from build123d import *

# Parameters (mm, degrees)
SKETCH1_W               = 21
SKETCH1_H               = 9
BOSS_EXTRUDE1_DEPTH     = 4
CUT_EXTRUDE1_REACH      = 15.946
SKETCH2_W               = 17
SKETCH2_H               = 7
CUT_EXTRUDE3_REACH      = 15.946
SKETCH5_W               = 2
SKETCH5_H               = 9
BOSS_EXTRUDE2_REACH     = 21.931
SKETCH9_W               = 2
SKETCH9_H               = 3
BOSS_EXTRUDE3_DEPTH     = 8
SKETCH11_W              = 3
SKETCH11_H              = 5
BOSS_EXTRUDE4_DEPTH     = 11.25
BOSS_EXTRUDE5_START     = -4
BOSS_EXTRUDE5_OUTLINE_W = 3
BOSS_EXTRUDE5_OUTLINE_H = 5
BOSS_EXTRUDE5_DEPTH     = 8
SKETCH13_R              = 0.75
CUT_EXTRUDE4_DEPTH      = 2.5
BOSS_EXTRUDE6_DEPTH     = 5
BOSS_EXTRUDE7_REACH     = 29.795


# Read off the part's stored shape, not the designer's step: Boss-Extrude5
with BuildPart() as part:
    # Sketch1 → Boss-Extrude1 (new, symmetric)
    with BuildSketch(Plane.XY):
        Rectangle(SKETCH1_W, SKETCH1_H)
    extrude(amount=BOSS_EXTRUDE1_DEPTH, both=True)

    # Sketch2 → Cut-Extrude1 (cut, up to next)
    with BuildSketch(Plane.XY.offset(4), mode=Mode.PRIVATE) as cut_extrude1_sk1:
        with Locations((0, -1)):
            Rectangle(SKETCH2_W, SKETCH2_H)
    cut_extrude1_tool1 = extrude(cut_extrude1_sk1.sketch, amount=-CUT_EXTRUDE1_REACH, mode=Mode.PRIVATE) & part.part
    add(cut_extrude1_tool1.solids().sort_by_distance((0, -1, 4))[0], mode=Mode.SUBTRACT)

    # Sketch5 → Cut-Extrude3 (cut, up to next)
    with BuildSketch(Plane.XY.offset(4), mode=Mode.PRIVATE) as cut_extrude3_sk1:
        with Locations((-9.5, 0)):
            Rectangle(SKETCH5_W, SKETCH5_H)
    cut_extrude3_tool1 = extrude(cut_extrude3_sk1.sketch, amount=-CUT_EXTRUDE3_REACH, mode=Mode.PRIVATE) & part.part
    add(cut_extrude3_tool1.solids().sort_by_distance((-9.5, 0, 4))[0], mode=Mode.SUBTRACT)

    # Sketch7 → Boss-Extrude2 (add, up to next)
    with BuildSketch(Plane.ZY.offset(8.5), mode=Mode.PRIVATE) as boss_extrude2_sk1:
        Polygon((1, 2.5), (-1, 2.5), (-1.75, 1), (1.75, 1), align=None)
    boss_extrude2_tool1 = extrude(boss_extrude2_sk1.sketch, amount=-BOSS_EXTRUDE2_REACH, mode=Mode.PRIVATE) - part.part
    add(boss_extrude2_tool1.solids().sort_by_distance((-8.5, 1.681818, 0))[0])

    # Sketch9 → Boss-Extrude3 (add)
    with BuildSketch(Plane.XY.offset(4)):
        with Locations((9.5, -6)):
            Rectangle(SKETCH9_W, SKETCH9_H)
    extrude(amount=-BOSS_EXTRUDE3_DEPTH)

    # Sketch11 → Boss-Extrude4 (add)
    with BuildSketch(Plane(origin=(10.5, 0, 0), x_dir=(0, 0, -1), z_dir=(1, 0, 0))):
        with Locations((0, -5)):
            Rectangle(SKETCH11_W, SKETCH11_H)
    extrude(amount=BOSS_EXTRUDE4_DEPTH)

    # Boss-Extrude5 outline → Boss-Extrude5 (add)
    with BuildSketch(Plane.XY.offset(BOSS_EXTRUDE5_START)):
        with Locations((23.25, -5)):
            Rectangle(BOSS_EXTRUDE5_OUTLINE_W, BOSS_EXTRUDE5_OUTLINE_H)
    extrude(amount=BOSS_EXTRUDE5_DEPTH)

    # Sketch13 → Cut-Extrude4 (cut)
    with BuildSketch(Plane(origin=(24.75, 0, 0), x_dir=(0, 0, -1), z_dir=(1, 0, 0))):
        with Locations((0, -4)):
            Circle(SKETCH13_R)
    extrude(amount=-CUT_EXTRUDE4_DEPTH, mode=Mode.SUBTRACT)

    # Sketch14 → Boss-Extrude6 (add)
    with BuildSketch(Plane.XZ.offset(7.5)):
        Polygon((21.75, 4), (20.306624327, 1.5), (21.75, 1.5), align=None)
        Polygon((21.75, -4), (21.75, -1.5), (20.306624327, -1.5), align=None)
    extrude(amount=-BOSS_EXTRUDE6_DEPTH)

    # Boss-Extrude7: up to this face of the body (flat: up to its plane)
    boss_extrude7_end = Plane(part.part.faces().sort_by_distance((1, 4.5, 0))[0])
    # Sketch15 → Boss-Extrude7 (add, up to the picked face)
    with BuildSketch(Plane.XZ.offset(7.5), mode=Mode.PRIVATE) as boss_extrude7_sk1:
        Polygon((8.5, 4), (8.5, -4), (6.190598923, 0), align=None)
    boss_extrude7_tool1 = split(extrude(boss_extrude7_sk1.sketch, amount=-BOSS_EXTRUDE7_REACH, mode=Mode.PRIVATE), bisect_by=boss_extrude7_end, keep=Keep.BOTH, mode=Mode.PRIVATE)
    add(boss_extrude7_tool1.solids().sort_by(Axis((7.7302, -7.5, 0), (0, 1, 0)))[0])


solid = part.part
Part model, mm, in its own coordinate system. A direction names the side the tool comes from. Coordinates: 2 decimals unless noted, no trailing zeros. Order: outer loops, then holes, each group sorted by start corner. A loop starts at its lowest first (then second) coordinate and runs counter-clockwise, first axis right, second up. Notation, with made-up numbers: (-35.75, 73.5) - (-26.75, 73.5) arc R27 ccw to (-26.75, 93.5) - close; hole circle Ø2 at (73, -15). An arc over 180 degrees is marked (long way). Use CSV: the item, a comma, the result in double quotes.
Item 1: Drop flat-ended pins along their axis: P1, Ø6, axis at x = 17.5, y = 3, coming from the -Z side; P2, Ø1.2, axis at y = -4, z = 0, coming from the +X side; P3, Ø2.5, axis at x = 17, y = -6, coming from the +Z side; P4, Ø3.5, axis at x = -1.5, z = -3, coming from the -Y side. Give the stop position or say it passes through.
Solved:
P1,"passes through"
P2,"stops at x = 22.25"
P3,"stops at z = 1.5"
P4,"stops at y = 1"
Item 2: Saw through at C-C on y = -6.25. Give the cut face in (x, z), and give its area (3 significant figures).
Solved:
outline,"(6.19, 0) - (8.5, -4) - (10.5, -4) - (10.5, -1.5) - (20.31, -1.5) - (21.75, -4) - (24.75, -4) - (24.75, 4) - (21.75, 4) - (20.31, 1.5) - (10.5, 1.5) - (10.5, 4) - (8.5, 4) - close"
area,"86.6 mm²"
Item 3: Saw through at B-B on z = 2.75. Give the cut face in (x, y).
Solved:
outline,"(-8.5, 2.5) - (7.78, 2.5) - (7.78, -7.5) - (10.5, -7.5) - (10.5, 4.5) - (-8.5, 4.5) - close; (21.03, -7.5) - (24.75, -7.5) - (24.75, -2.5) - (21.03, -2.5) - close"
Item 4: 3-axis set-ups, long thin cutter, end or side, ignore diameter. For faces 1 (the face through (10.5, -2, 0)), 2 (the face through (22.25, -4, 0)), 3 (the face through (15, -5, -1.5)): which of +Z, -Z, +X, -X, +Y, -Y reach the whole face in a straight line?
Solved:
face 1,"+Y"
face 2,"+X"
face 3,"-Z, +Y, -Y"
Item 5: Probe probe 1 along Y at (x, z) = (23.5, 0); probe 2 along Z at (x, y) = (20, -5.25); probe 3 along X at (y, z) = (1.25, -1.75). List the from-to ranges inside material, lowest first.
Solved:
probe 1,"y = -7.5 to -4.75, -3.25 to -2.5"
probe 2,"z = -1.5 to 1.5"
probe 3,"x = 7.2 to 10.5"
Item 6: Saw through at A-A on y = -4. Give the cut face in (x, z), and give its area (3 significant figures).
Solved:
outline,"(6.19, 0) - (8.5, -4) - (10.5, -4) - (10.5, -1.5) - (20.31, -1.5) - (21.75, -4) - (24.75, -4) - (24.75, -0.75) - (22.25, -0.75) - (22.25, 0.75) - (24.75, 0.75) - (24.75, 4) - (21.75, 4) - (20.31, 1.5) - (10.5, 1.5) - (10.5, 4) - (8.5, 4) - close"
area,"82.8 mm²"
Item 7: Saw through at D-D on x = 16. Give the cut face in (y, z), and give its area (3 significant figures).
Solved:
outline,"(-7.5, -1.5) - (-2.5, -1.5) - (-2.5, 1.5) - (-7.5, 1.5) - close"
area,"15.0 mm²"
Item 8: Mould opens along X. For faces 4 (the face through (21, -5, -2.7)), 5 (the face through (-8.5, 3, 0)), 6 (the face through (23, -5, -4)), 7 (the face through (24.75, -5, 0)) say: +X half, -X half, draft (parallel to the pull), parting line (faces both ways), or undercut.
Solved:
face 4,"undercut"
face 5,"-X half"
face 6,"draft"
face 7,"+X half"
